```python
from build123d import *

# Parameters (mm, degrees)
SKETCH1_W           = 6.35
SKETCH1_H           = 101.6
BOSS_EXTRUDE1_DEPTH = 457.2
SKETCH2_R           = 12.7
CUT_EXTRUDE1_DEPTH  = 467.602190566
SKETCH3_W           = 9.117948718
SKETCH3_H           = 50.8
CUT_EXTRUDE2_DEPTH  = 467.602190566


with BuildPart() as part:
    # Sketch1 → Boss-Extrude1 (new body)
    with BuildSketch(Plane(origin=(0, 0, 0), x_dir=(0, 0, -1), z_dir=(1, 0, 0))):
        with Locations((1.913371748, -42.180867605)):
            Rectangle(SKETCH1_W, SKETCH1_H)
    extrude(amount=BOSS_EXTRUDE1_DEPTH)

    # Sketch2 → Cut-Extrude1 (cut, through all)
    with BuildSketch(Plane(origin=(0, 0, -5.088371748), x_dir=(-1, 0, 0), z_dir=(0, 0, -1))):
        with Locations(Location((-355.6, -42.180867605, 0), (0, 0, 90))):
            Circle(SKETCH2_R)
        with Locations(Location((-101.6, -42.180867605, 0), (0, 0, 90))):
            Circle(SKETCH2_R)
    extrude(amount=-CUT_EXTRUDE1_DEPTH, mode=Mode.SUBTRACT)

    # Sketch3 → Cut-Extrude2 (cut, through all)
    with BuildSketch(Plane(origin=(0, 0, -5.088371748), x_dir=(-1, 0, 0), z_dir=(0, 0, -1))):
        with BuildLine():
            Line((-438.15, -4.080867605), (-402.680256121, -4.080867605))
            ThreePointArc((-402.680256121, -4.080867605), (-396.81362109, -8.000827809), (-398.190128061, -14.920995665))
            Line((-398.190128061, -14.920995665), (-433.659871939, -50.390739544))
            ThreePointArc((-433.659871939, -50.390739544), (-440.580039796, -51.767246515), (-444.5, -45.900611484))
            Line((-444.5, -45.900611484), (-444.5, -10.430867605))
            ThreePointArc((-444.5, -10.430867605), (-442.640128061, -5.940739544), (-438.15, -4.080867605))
        make_face()
        with BuildLine():
            Line((-398.190128061, -33.970995665), (-433.659871939, -69.440739544))
            ThreePointArc((-433.659871939, -69.440739544), (-435.03637891, -76.3609074), (-429.169743879, -80.280867605))
            Line((-429.169743879, -80.280867605), (-393.7, -80.280867605))
            ThreePointArc((-393.7, -80.280867605), (-389.209871939, -78.420995665), (-387.35, -73.930867605))
            Line((-387.35, -73.930867605), (-387.35, -38.461123726))
            ThreePointArc((-387.35, -38.461123726), (-391.269960204, -32.594488694), (-398.190128061, -33.970995665))
        make_face()
        with BuildLine():
            Line((-69.85, -73.930867605), (-69.85, -38.461123726))
            ThreePointArc((-69.85, -38.461123726), (-65.930039796, -32.594488694), (-59.009871939, -33.970995665))
            Line((-59.009871939, -33.970995665), (-23.540128061, -69.440739544))
            ThreePointArc((-23.540128061, -69.440739544), (-22.16362109, -76.3609074), (-28.030256121, -80.280867605))
            Line((-28.030256121, -80.280867605), (-63.5, -80.280867605))
            ThreePointArc((-63.5, -80.280867605), (-67.990128061, -78.420995665), (-69.85, -73.930867605))
        make_face()
        with BuildLine():
            Line((-23.540128061, -50.390739544), (-59.009871939, -14.920995665))
            ThreePointArc((-59.009871939, -14.920995665), (-60.38637891, -8.000827809), (-54.519743879, -4.080867605))
            Line((-54.519743879, -4.080867605), (-19.05, -4.080867605))
            ThreePointArc((-19.05, -4.080867605), (-14.559871939, -5.940739544), (-12.7, -10.430867605))
            Line((-12.7, -10.430867605), (-12.7, -45.900611484))
            ThreePointArc((-12.7, -45.900611484), (-16.619960204, -51.767246515), (-23.540128061, -50.390739544))
        make_face()
        Polygon((-317.614703405, -17.01094408), (-290.260857251, -17.01094408), (-290.260857251, -26.128892798), (-299.378805969, -26.128892798), (-299.378805969, -67.81094408), (-308.496754687, -67.81094408), (-308.496754687, -26.128892798), (-317.614703405, -26.128892798), align=None)
        Polygon((-283.096754687, -17.01094408), (-255.742908533, -17.01094408), (-255.742908533, -26.128892798), (-273.978805969, -26.128892798), (-273.978805969, -35.898123567), (-255.742908533, -35.898123567), (-255.742908533, -45.016072285), (-273.978805969, -45.016072285), (-273.978805969, -58.692995362), (-255.742908533, -58.692995362), (-255.742908533, -67.81094408), (-283.096754687, -67.81094408), align=None)
        Polygon((-250.858293149, -17.01094408), (-241.119591226, -17.01094408), (-228.063421354, -53.096040233), (-214.976722636, -17.01094408), (-205.268549559, -17.01094408), (-223.687620072, -67.81094408), (-232.469751482, -67.81094408), align=None)
        with Locations((-193.871113661, -42.41094408)):
            Rectangle(SKETCH3_W, SKETCH3_H)
        Polygon((-177.589062379, -17.01094408), (-169.376802764, -17.01094408), (-146.327523918, -50.440030618), (-146.327523918, -17.01094408), (-137.2095752, -17.01094408), (-137.2095752, -67.81094408), (-145.482892508, -67.81094408), (-168.471113661, -34.483620362), (-168.471113661, -67.81094408), (-177.589062379, -67.81094408), align=None)
    extrude(amount=-CUT_EXTRUDE2_DEPTH, mode=Mode.SUBTRACT)


solid = part.part
```
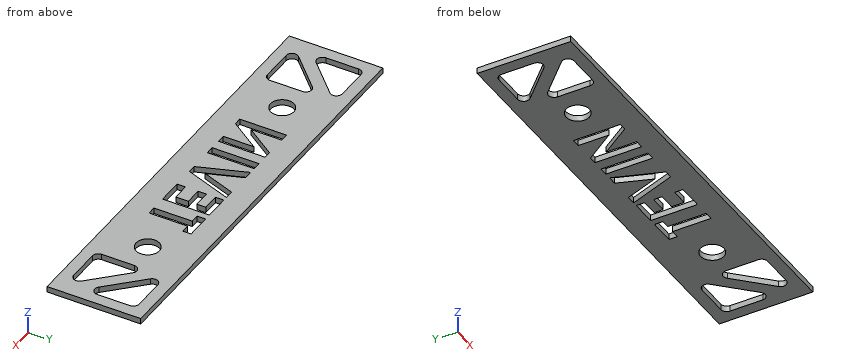
Geometry check sheet. Reference: the model listing, model coordinates, mm. Coordinates: 2 decimals unless noted, no trailing zeros. Order: outer loops, then holes, each group sorted by start corner. A loop starts at its lowest first (then second) coordinate and runs counter-clockwise, first axis right, second up.
Item 1: Section check A-A (x = 355.6). Enter the section's corners in (y, z).
Item 2: Section check C-C (x = 278). Enter the section's corners in (y, z), plus the area to 3 significant figures.
Item 3: Section check B-B (z = -1). Count the separate pieces of the cut face and the enclosed holes in it, plus the area to 3 significant figures.
Item 4: Scan lines: line 1 along X through (y, z) = (-74, -1.75); line 2 along Y through (x, z) = (415, 0.5); line 3 along Y through (x, z) = (402, -4). Record each from-to range of solid material in increasing order.
Check sheet entries:
1. outline: (-92.98, -5.09) - (-54.88, -5.09) - (-54.88, 1.26) - (-92.98, 1.26) - close; (-29.48, -5.09) - (8.62, -5.09) - (8.62, 1.26) - (-29.48, 1.26) - close
2. outline: (-92.98, -5.09) - (-67.81, -5.09) - (-67.81, 1.26) - (-92.98, 1.26) - close; (-17.01, -5.09) - (8.62, -5.09) - (8.62, 1.26) - (-17.01, 1.26) - close
2. area: 323 mm2
3. separate pieces: 1
3. enclosed holes: 11
3. area: 35,100 mm2
4. line 1: x = 0 to 21.68, 69.85 to 387.35, 435.52 to 457.2
4. line 2: y = -92.98 to -80.28, -50.78 to -31.73, -4.08 to 8.62
4. line 3: y = -92.98 to -80.28, -37.78 to -18.73, -4.12 to 8.62
